Here's how the part is built. I have some questions about the finished solid (model axes, mm). A direction names the side the tool comes from. Round coordinates to 2 decimals unless told otherwise and drop trailing zeros. Write each loop counter-clockwise with the first axis right and the second up, starting at its lowest first coordinate (ties: lowest second). Pieces come first, ordered by that corner, then holes. Notation, with made-up numbers: (51, 3) -> (58, 3) arc R12 ccw to (58, 8) -> close; hole circle Ø1 at (41.5, -8). An arc over 180 degrees is marked (long way). Answer in a Markdown table with one row per item.
from build123d import *

# Parameters (mm, degrees)
F1_DEPTH      = 60.325
F2_R          = 12.7
F3_DEPTH      = 60.326
F4_DEPTH      = 19.05
F5_W          = 37.9222
F5_H          = 41.275
F6_DEPTH      = 34.798
F7_R          = 6.35
F7_W          = 53.7857485574
F7_H          = 22.3266
F8_DEPTH      = 9.5573214296
F8_DEPTH_BACK = 47.5946785704


with BuildPart() as f1:
    # F0 (on Front) → F1 (new body)
    with BuildSketch(Plane.XZ):
        with BuildLine():
            ThreePointArc((-68.6650304641, 12.7956785704), (-71.9075169357, 13.9650927471), (-73.6571649634, 16.9349378297))
            ThreePointArc((-73.6571649634, 16.9349378297), (-112.8291343827, 27.0626190455), (-95.6225567601, -9.5563214296))
            Line((-95.6225567601, -9.5563214296), (98.5858432399, -9.5563214296))
            Line((98.5858432399, -9.5563214296), (98.5858432399, 4.9216785704))
            ThreePointArc((98.5858432399, 4.9216785704), (96.279602035, 10.4894373655), (90.7118432399, 12.7956785704))
            Line((90.7118432399, 12.7956785704), (59.5460432399, 12.7956785704))
            ThreePointArc((59.5460432399, 12.7956785704), (55.9539407915, 14.283576122), (54.4660432399, 17.8756785704))
            Line((54.4660432399, 17.8756785704), (54.4660432399, 42.5136785704))
            ThreePointArc((54.4660432399, 42.5136785704), (52.9781456883, 46.1057810189), (49.3860432399, 47.5936785704))
            Line((49.3860432399, 47.5936785704), (35.4160432399, 47.5936785704))
            ThreePointArc((35.4160432399, 47.5936785704), (31.8418586015, 28.8780362045), (21.6238432399, 12.7956785704))
            Line((21.6238432399, 12.7956785704), (-68.6650304641, 12.7956785704))
        make_face()
    extrude(amount=F1_DEPTH)

    # F2 (on face) → F3 (cut, through all)
    with BuildSketch(Plane.XZ.offset(60.325)):
        with Locations((-95.6225567601, 12.7956785704)):
            Circle(F2_R)
    extrude(amount=-F3_DEPTH, mode=Mode.SUBTRACT)

    # F2 (on face) → F4 (cut)
    with BuildSketch(Plane.XZ.offset(60.325)):
        Polygon((21.6238432399, 12.7956785704), (-9.7705567601, 12.7956785704), (-3.7761567601, -9.5563214296), (21.6238432399, -9.5563214296), align=None)
    extrude(amount=-F4_DEPTH, mode=Mode.SUBTRACT)

    # F5 (on face) → F6 (cut)
    with BuildSketch(Plane.XY.offset(47.5936785704)):
        with Locations((40.5849432399, -20.6375)):
            Rectangle(F5_W, F5_H)
    extrude(amount=-F6_DEPTH, mode=Mode.SUBTRACT)

    # F7 (on Top) → F8 (cut, two sides)
    with BuildSketch(Plane.XY) as f8_sk:
        with Locations((59.7238432399, -22.352)):
            Circle(F7_R)
        with Locations((-91.0816824814, -30.1625)):
            Rectangle(F7_W, F7_H)
    extrude(amount=-F8_DEPTH, mode=Mode.SUBTRACT)
    extrude(f8_sk.sketch, amount=F8_DEPTH_BACK, mode=Mode.SUBTRACT)


solid = f1.part
1) I want a section at A-A, the plane y = -44. List the corners of the cut face in (x, z) for me, and give its area (3 significant figures).
Response:
| item | result |
|---|---|
| outline | (-95.62, -9.56) -> (-3.78, -9.56) -> (-9.77, 12.8) -> (-68.67, 12.8) arc R5.08 cw to (-73.66, 16.93) arc R22.35 ccw (long way) to start; (21.62, -9.56) -> (98.59, -9.56) -> (98.59, 4.92) arc R7.87 ccw to (90.71, 12.8) -> (59.55, 12.8) arc R5.08 cw to (54.47, 17.88) -> (54.47, 42.51) arc R5.08 ccw to (49.39, 47.59) -> (35.42, 47.59) arc R50.8 cw to (21.62, 12.8) -> close; hole circle Ø25.4 at (-95.62, 12.8) |
| area | 5,180 mm^2 |
2) I want a section at B-B, the plane y = -8. List the corners of the cut face in (x, z) for me, and give its area (3 significant figures).
Response:
| item | result |
|---|---|
| outline | (-95.62, -9.56) -> (98.59, -9.56) -> (98.59, 4.92) arc R7.87 ccw to (90.71, 12.8) -> (-68.67, 12.8) arc R5.08 cw to (-73.66, 16.93) arc R22.35 ccw (long way) to start; hole circle Ø25.4 at (-95.62, 12.8) |
| area | 5,000 mm^2 |
3) I want a section at D-D, the plane z = 27.5. List the corners of the cut face in (x, y) for me (3 decimals).
Response:
| item | result |
|---|---|
| outline | (-112.457, -60.325) -> (-78.788, -60.325) -> (-78.788, -41.326) -> (-112.457, -41.326) -> close; (-112.457, -18.999) -> (-78.788, -18.999) -> (-78.788, 0) -> (-112.457, 0) -> close; (31.272, -60.325) -> (54.466, -60.325) -> (54.466, -41.275) -> (31.272, -41.275) -> close |
4) For pin 1 (12 mm diameter, centred on y = -47, z = -3.5, fed in from -X); pin 2 (1.5 mm diameter, centred on y = -42, z = 23.5, fed in from +X); pin 3 (4 mm diameter, centred on x = 51.5, y = -26, fed in from +Z), each with a flat end and sliding along its axis, tell me the tip position at first contact or that it passes through.
Response:
| item | result |
|---|---|
| pin 1 | stops at x = -115.46 |
| pin 2 | stops at x = 54.47 |
| pin 3 | stops at z = 12.8 |
5) I need wall thicknesses on line 1 (Y direction, x = -81, z = 17) (3 decimals); line 2 (Y direction, x = -4, z = 4) (3 decimals); line 3 (X direction, y = -35, z = -6). Which ranges of each line are inside material? Lowest first, please. Write a range as [from, to].
Response:
| item | result |
|---|---|
| line 1 | y = [-60.325, -41.326], [-18.999, 0] |
| line 2 | y = [-41.275, 0] |
| line 3 | x = [-64.19, 98.59] |
6) I want a section at C-C, the plane x = 44.5. List the corners of the cut face in (y, z) for me (3 decimals), and give its area (3 significant figures).
Response:
| item | result |
|---|---|
| outline | (-60.325, -9.556) -> (0, -9.556) -> (0, 12.796) -> (-41.275, 12.796) -> (-41.275, 47.594) -> (-60.325, 47.594) -> close |
| area | 2,010 mm^2 |
7) Which directions (+Z, -Z, +X, -X, +Y, -Y) give clear straight access to the entire face, cutting with the end or side of a thin tool? Please do faces 4 (the face through (54.466, -51, 30)), 5 (the face through (45, -41.275, 30)), 6 (the face through (-85, -41.326, 3)).
Response:
| item | result |
|---|---|
| face 4 | +Z, +X, +Y, -Y |
| face 5 | +Z, +X, -X, +Y |
| face 6 | +Z, -Z, -X |
8) We'd pull the mould along X, two halves only. Please class faces 1 (the face through (31.94, -50.67, 29.13)), 2 (the face through (98.586, -30, -2)), 3 (the face through (-62, -60.325, 8)): +X half, -X half, draft (parallel to the pull), parting line (faces both ways), or undercut.
Response:
| item | result |
|---|---|
| face 1 | undercut |
| face 2 | +X half |
| face 3 | draft |
